Autodesk Inventor part; units mm, degrees
ref_plane "YZ Plane" through (0, 0, 0) normal (1, 0, 0) x (0, 1, 0)
ref_plane "XZ Plane" through (0, 0, 0) normal (0, 1, 0) x (-1, 0, 0)
ref_plane "XY Plane" through (0, 0, 0) normal (0, 0, 1) x (1, 0, 0)
ref_plane "Arbeitsebene1" through (-1.9028, 0, 2) normal (0, 0, 1) x (-0.2882, -0.9576, 0)
sketch "Skizze1" plane through (-1.9028, 0, 2) normal (0, 0, 1) x (-0.2882, -0.9576, 0)
  circle A0 centre (-14.632, 0) radius 18.75
  circle A1 centre (-14.632, 0) radius 15
  circle A2 centre (-14.632, 0) radius 16.2815
  line L0 (26.7708, -9) -> (26.7708, -29)
  line L1 (19.0208, -9) -> (26.7708, -9)
  line L2 (26.7708, -29) -> (19.0208, -29)
  line L3 (27.1135, -8.6759) -> (1.6495, -8.6759)
  line L4 (1.6495, -8.6759) -> (1.6495, 0)
  line L5 (1.6495, 0) -> (27.1135, 0)
  line L6 (27.1135, 0) -> (27.1135, -8.6759)
  point P0 (-12.7292, 0)
extrude "Extrusion1" add sketch "Skizze1" along normal blind 5 contours L5 L4 L3 A0 | L5 L6 L3 A0 | A0 L3 L4 L5
properties part number "15_Gabel"
Part model, mm, in its own coordinate system. Coordinates: 2 decimals unless noted, no trailing zeros. Write each loop counter-clockwise with the first axis right and the second up, starting at its lowest first coordinate (ties: lowest second). Pieces come first, ordered by that corner, then holes.
Item 1: Probe line 1 (X direction, y = 19, z = 4.25); line 2 (X direction, y = 4.5, z = 2.9); line 3 (Y direction, x = -10, z = 4.2). List the from-to ranges inside material, lowest first.
Item 2: Slice it at B-B (y = 17). Write the cut outline in (x, z), and give its area (3 significant figures).
Item 3: Slice it at A-A (x = -15). Write the cut outline in (y, z), and give its area (3 significant figures).
Item 4: Slice it at D-D (y = -13). Write the cut outline in (x, z), and give its area (3 significant figures).
Item 5: Mould opens along X. For faces 1 (the face through (-7, 0, 7)), 2 (the face through (6.316, 29.793, 4.465)), 3 (the face through (-14.455, -11.602, 4.465)) say: released by +X, released by -X, zero draft, split by the parting line, or undercut.
Results found:
1. line 1: x = -15.76 to -13.18, 17.81 to 20.39
1. line 2: x = -13.84 to -10.9, 15.53 to 18.47
1. line 3: y = -25.88 to 3.36, 24.66 to 28.15
2. outline: (-16.2, 2) - (-13.69, 2) - (-13.69, 7) - (-16.2, 7) - close; (18.32, 2) - (20.82, 2) - (20.82, 7) - (18.32, 7) - close
2. area: 25.1 mm2
3. outline: (-24.37, 2) - (-13.41, 2) - (-13.41, 7) - (-24.37, 7) - close; (6.81, 2) - (21.21, 2) - (21.21, 7) - (6.81, 7) - close
3. area: 127 mm2
4. outline: (-14.88, 2) - (-5.82, 2) - (-5.82, 7) - (-14.88, 7) - close
4. area: 45.3 mm2
5. face 1: zero draft
5. face 2: undercut
5. face 3: released by -X
